Geometry: final body of the model. Coordinates: model frame, mm. Face numbers are marked on the shaded views. A direction names the side the tool comes from. Coordinates: 2 decimals unless noted, no trailing zeros. Loops run counter-clockwise (first coordinate to the right, second up) from the corner with the lowest first, then second, coordinate; pieces in that order, holes last. Notation, with made-up numbers: (57, 63) -> (78, 63) arc R18 ccw to (78, 68) -> close; hole circle Ø3 at (-11.5, 24.25). An arc over 180 degrees is marked (long way). One line per item, written item: value. Start each with the question number.
Item 1: Section query A-A on x = 42. Return loops of the section in (y, z), then the cut area to 3 significant figures.
Item 2: Section query C-C on y = -30.5. Return loops of the section in (x, z), then the cut area to 3 significant figures.
Item 3: Ray query, probe 1 along Y at (x, z) = (16.5, 0.75); probe 2 along X at (y, z) = (14.5, 1); probe 3 along Z at (x, y) = (-26, 12). Return the intervals inside material, ascending. Write a range as from..to.
Item 4: Section query B-B on y = 10.5. Return loops of the section in (x, z).
Item 5: Set-up query: the marked faces 1, 2 and 3. Return all of +Z, -Z, +X, -X, +Y, -Y with unobstructed straight access to the full face (end or side cutting, diameter ignored); none if empty.
Item 6: Section query D-D on y = -8.5. Return loops of the section in (x, z).
Item 7: Contact query for flat-ended pins moving along their axis: pin 1 Ø6 at (x, z) = (7, -3.5) entering from -Y; pin 2 Ø6.5 at (y, z) = (-28, 2) entering from -X; pin 3 Ø8.5 at (x, y) = (41.38, 12.34) entering from -Z. Output: stop coordinate, or through.
from build123d import *

# Parameters (mm, degrees)
F0_W          = 101.4095
F0_H          = 43.5991
F1_DEPTH      = 2.794
F2_R          = 6.6548
F2_R_2        = 3.8608
F3_DEPTH      = 23.71725
F3_DEPTH_BACK = 23.71725
F5_D          = 7.3533
F5_DEPTH      = 12.7


with BuildPart() as f1:
    # F0 (on Top) → F1 (new body)
    with BuildSketch(Plane.XY):
        with Locations((0.00635, 0)):
            Rectangle(F0_W, F0_H)
    extrude(amount=F1_DEPTH)

    # F2 (on Right) → F3 (join, two sides)
    with BuildSketch(Plane.YZ) as f3_sk:
        with Locations((-28.306066, 1.397)):
            Circle(F2_R)
        with Locations((-28.306066, 1.397)):
            Circle(F2_R_2, mode=Mode.SUBTRACT)
    extrude(amount=F3_DEPTH)
    extrude(f3_sk.sketch, amount=-F3_DEPTH_BACK)

    # F5
    with Locations(Plane.XY.offset(2.794)):
        with Locations((14.0208, 4.10845), (-14.0081, 12.33805), (-41.3639, 4.10845), (41.3766, 12.33805)):
            Hole(F5_D / 2, depth=F5_DEPTH)


solid = f1.part
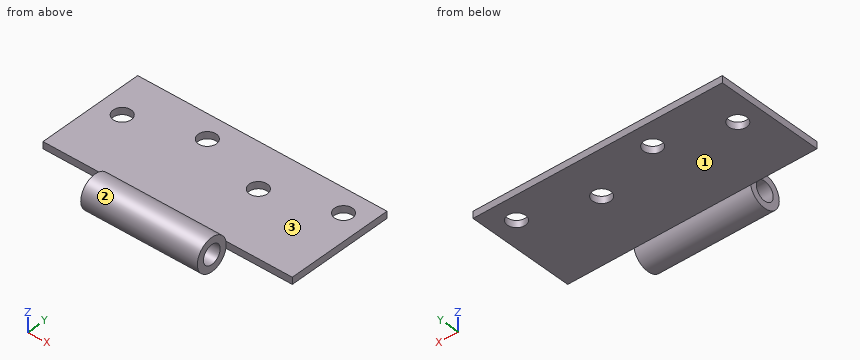
Reply:
1. outline: (-21.8, 0) -> (8.71, 0) -> (8.71, 2.79) -> (-21.8, 2.79) -> close; (15.96, 0) -> (21.8, 0) -> (21.8, 2.79) -> (15.96, 2.79) -> close
1. area: 102 mm²
2. outline: (-23.72, -4.89) -> (23.72, -4.89) -> (23.72, -1.78) -> (-23.72, -1.78) -> close; (-23.72, 4.57) -> (23.72, 4.57) -> (23.72, 7.68) -> (-23.72, 7.68) -> close
2. area: 295 mm²
3. probe 1: y = -34.93..-32.11, -24.5..1.39, 6.82..21.8
3. probe 2: x = -50.7..-16.98, -11.03..38.4, 44.35..50.71
3. probe 3: z = 0..2.79
4. outline: (-50.7, 0) -> (-17.19, 0) -> (-17.19, 2.79) -> (-50.7, 2.79) -> close; (-10.82, 0) -> (38.19, 0) -> (38.19, 2.79) -> (-10.82, 2.79) -> close; (44.56, 0) -> (50.71, 0) -> (50.71, 2.79) -> (44.56, 2.79) -> close
5. face 1: -Z, +X, -X, +Y
5. face 2: +X, -X
5. face 3: +Z, +X, -X, +Y
6. outline: (-50.7, 0) -> (50.71, 0) -> (50.71, 2.79) -> (-50.7, 2.79) -> close
7. pin 1: stops at y = -34.68
7. pin 2: stops at x = -23.72
7. pin 3: stops at z = 0
